Source: CAD feature listing. Evaluate the final solid. Frame: model axes, mm. A direction names the side the tool comes from. Give positions to 0.01 mm unless a question says otherwise; leave off trailing zeros. Order: outer loops, then holes, each group sorted by start corner. A loop starts at its lowest first (then second) coordinate and runs counter-clockwise, first axis right, second up. Notation, with made-up numbers: (81, 13.5) -> (133, 13.5) arc R16 cw to (133, 29.5) -> close; hole circle Ø2 at (-24, -15). An arc over 180 degrees is marked (long way). Use CSV: the item, a comma, the result in double quotes.
```python
from build123d import *

# Parameters (mm, degrees)
SKETCH_1_W          = 66
SKETCH_1_H          = 25
EXTRUDE_1_DEPTH     = 3
SKETCH_2_W          = 3
SKETCH_2_H          = 25
EXTRUDE_2_DEPTH     = 35
SKETCH_3_R          = 1.5
CUT_EXTRUDE_1_DEPTH = 79.778169565


with BuildPart() as part:
    # 草图1 → 凸台-拉伸1 (new body)
    with BuildSketch(Plane.XY):
        with Locations((33, -12.5)):
            Rectangle(SKETCH_1_W, SKETCH_1_H)
    extrude(amount=EXTRUDE_1_DEPTH)

    # 草图2 → 凸台-拉伸2 (add)
    with BuildSketch(Plane(origin=(0, 0, 0), x_dir=(-1, 0, 0), z_dir=(0, 0, -1))):
        with Locations((-1.5, -12.5)):
            Rectangle(SKETCH_2_W, SKETCH_2_H)
        with Locations((-64.5, -12.5)):
            Rectangle(SKETCH_2_W, SKETCH_2_H)
    extrude(amount=EXTRUDE_2_DEPTH)

    # 草图3 → 切除-拉伸1 (cut, through all)
    with BuildSketch(Plane.ZY):
        with Locations(Location((-25, -6.25, 0), (0, 0, 270))):
            Circle(SKETCH_3_R)
        with Locations((-25, -18.75)):
            Circle(SKETCH_3_R)
    extrude(amount=-CUT_EXTRUDE_1_DEPTH, mode=Mode.SUBTRACT)


solid = part.part
```
1. Mould query, pull axis Z, two halves, no side actions, for faces 1 (the flat face through (33, -12, 3)), 2 (the flat face through (33, -12, 0)), 3 (the flat face through (66, -13, -16)), 4 (the cylindrical face through (64.479, -6.055, -23.513)). Classes: released by +Z, released by -Z, zero draft, split by the parting line, or undercut.
Answer below:
face 1,"released by +Z"
face 2,"released by -Z"
face 3,"zero draft"
face 4,"undercut"
2. Pin query (flat end, axial travel): P1, Ø12.5, axis at x = 20, y = -18, coming from the -Z side; P2, Ø2.5, axis at y = -6.25, z = -25, coming from the -X side. Return the tip coordinate at first contact, or that it passes through.
Answer below:
P1,"stops at z = 0"
P2,"passes through"
3. Ray query, line 1 along X through (y, z) = (-5, -13); line 2 along Z through (x, y) = (1.3, -6.25); line 3 along Z through (x, y) = (40, -16). Return the intervals inside material, ascending.
Answer below:
line 1,"x = 0 to 3, 63 to 66"
line 2,"z = -35 to -26.5, -23.5 to 3"
line 3,"z = 0 to 3"
4. Section query C-C on z = -25. Return loops of the section in (x, y), plus the area to 3 significant figures.
Answer below:
outline,"(0, -25) -> (3, -25) -> (3, -20.25) -> (0, -20.25) -> close; (0, -17.25) -> (3, -17.25) -> (3, -7.75) -> (0, -7.75) -> close; (0, -4.75) -> (3, -4.75) -> (3, 0) -> (0, 0) -> close; (63, -25) -> (66, -25) -> (66, -20.25) -> (63, -20.25) -> close; (63, -17.25) -> (66, -17.25) -> (66, -7.75) -> (63, -7.75) -> close; (63, -4.75) -> (66, -4.75) -> (66, 0) -> (63, 0) -> close"
area,"114 mm²"
5. Access query for faces 5 (the flat face through (36, -25, 1)), 6 (the flat face through (3, -13, -17)). Directions: +Z, -Z, +X, -X, +Y, -Y. A direction counts if a zero-diameter tool reaches every point of the face in a straight line with its end or side. Return the directions, or none.
Answer below:
face 5,"+Z, -Z, +X, -X, -Y"
face 6,"-Z, +Y, -Y"
6. Section query B-B on y = -18.75. Return loops of the section in (x, z).
Answer below:
outline,"(0, -35) -> (3, -35) -> (3, -26.5) -> (0, -26.5) -> close; (0, -23.5) -> (3, -23.5) -> (3, 0) -> (63, 0) -> (63, -23.5) -> (66, -23.5) -> (66, 3) -> (0, 3) -> close; (63, -35) -> (66, -35) -> (66, -26.5) -> (63, -26.5) -> close"
7. Section query A-A on z = -32. Return loops of the section in (x, y).
Answer below:
outline,"(0, -25) -> (3, -25) -> (3, 0) -> (0, 0) -> close; (63, -25) -> (66, -25) -> (66, 0) -> (63, 0) -> close"
8. Section query D-D on y = -3.5. Return loops of the section in (x, z).
Answer below:
outline,"(0, -35) -> (3, -35) -> (3, 0) -> (63, 0) -> (63, -35) -> (66, -35) -> (66, 3) -> (0, 3) -> close"
